from build123d import *

# Parameters (mm, degrees)
F1_DEPTH  = 25.4
F2_W      = 9.525
F2_H      = 19.05
F3_DEPTH  = 134.62
F4_W      = 9.525
F4_H      = 19.05
F5_DEPTH  = 157.48
F6_R      = 1.651
F7_DEPTH  = 25.4
F8_W      = 25.4
F8_H      = 7.62
F9_DEPTH  = 101.6
F10_W     = 15.24
F10_H     = 19.05
F10_W_2   = 25.4
F11_DEPTH = 25.4
F12_W     = 38.1
F12_H     = 18.161
F13_DEPTH = 25.4


with BuildPart() as f1:
    # F0 (on Top) → F1 (new body)
    with BuildSketch(Plane.XY):
        Polygon((125.723586, 125.723586), (0, 0), (152.4, 0), (152.4, 12.7), (31.75, 12.7), (135.248586, 116.198586), align=None)
    extrude(amount=F1_DEPTH)

    # F2 (on face) → F3 (cut)
    with BuildSketch(Plane.YZ.offset(152.4)):
        with Locations((7.9375, 12.7)):
            Rectangle(F2_W, F2_H)
    extrude(amount=-F3_DEPTH, mode=Mode.SUBTRACT)

    # F4 (on face) → F5 (cut)
    with BuildSketch(Plane(origin=(125.723586, 125.723586, 0), x_dir=(-0.707107, 0.707107, 0), z_dir=(0.707107, 0.707107, 0))):
        with Locations((-8.707884, 12.7)):
            Rectangle(F4_W, F4_H)
    extrude(amount=-F5_DEPTH, mode=Mode.SUBTRACT)

    # F6 (on face) → F7 (cut)
    with BuildSketch(Plane(origin=(0, 3.175, 0), x_dir=(-1, 0, 0), z_dir=(0, 1, 0))):
        with Locations((-88.9, 12.7)):
            Circle(F6_R)
        with Locations((-50.8, 12.7)):
            Circle(F6_R)
        with Locations((-127, 12.7)):
            Circle(F6_R)
    extrude(amount=-F7_DEPTH, mode=Mode.SUBTRACT)

    # F8 (on face) → F9 (cut)
    with BuildSketch(Plane.XY.offset(25.4)):
        with Locations((38.1, 6.35)):
            Rectangle(F8_W, F8_H)
        with Locations((69.85, 6.35)):
            Rectangle(F8_W, F8_H)
        with Locations((101.6, 6.35)):
            Rectangle(F8_W, F8_H)
        with Locations((133.35, 6.35)):
            Rectangle(F8_W, F8_H)
        Polygon((128.962406, 113.504509), (122.676227, 119.790688), (104.715715, 101.830176), (111.001894, 95.543997), align=None)
        Polygon((106.865048, 90.700587), (100.578869, 96.986766), (82.618356, 79.026254), (88.904536, 72.740075), align=None)
        Polygon((84.061126, 68.603228), (77.774947, 74.889408), (59.814434, 56.928895), (66.100614, 50.642716), align=None)
        Polygon((61.755537, 46.007537), (55.469357, 52.293716), (37.508845, 34.333204), (43.795024, 28.047025), align=None)
    extrude(amount=-F9_DEPTH, mode=Mode.SUBTRACT)

    # F10 (on face) → F11 (cut)
    with BuildSketch(Plane.XZ):
        with Locations((138.455176, 12.7)):
            Rectangle(F10_W, F10_H)
        with Locations((106.998765, 12.7)):
            Rectangle(F10_W_2, F10_H)
        with Locations((68.713241, 12.7)):
            Rectangle(F10_W_2, F10_H)
        with Locations((33.749367, 12.7)):
            Rectangle(F10_W_2, F10_H)
    extrude(amount=-F11_DEPTH, mode=Mode.SUBTRACT)

    # F12 (on face) → F13 (cut)
    with BuildSketch(Plane(origin=(0, 0, 0), x_dir=(-0.707107, -0.707107, 0), z_dir=(-0.707107, 0.707107, 0))):
        with Locations((-108.820044, 12.337992)):
            Rectangle(F12_W, F12_H)
        with Locations((-152.4, 12.337992)):
            Rectangle(F12_W, F12_H)
        with Locations((-64.913327, 12.337992)):
            Rectangle(F12_W, F12_H)
    extrude(amount=-F13_DEPTH, mode=Mode.SUBTRACT)


solid = f1.part
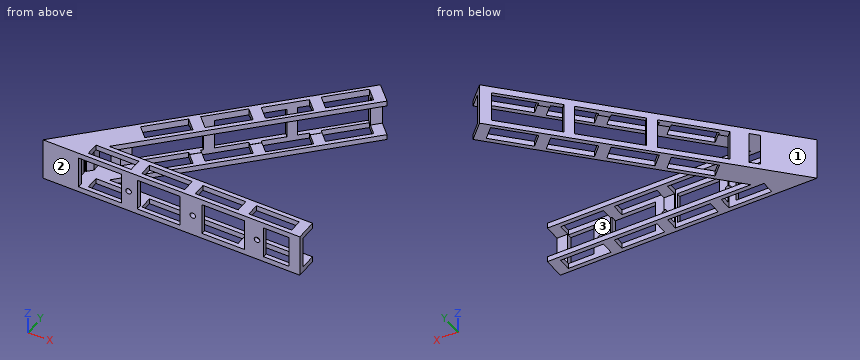
Geometry check sheet. Reference: the model listing, model coordinates, mm. Face numbers are marked on the shaded views. Coordinates: 2 decimals unless noted, no trailing zeros. Use a Markdown table: item, result. Add a question column.
1. Go/stop test with flat-tipped pins: pin 1 Ø3 at (y, z) = (17, 14) entering from +X; pin 2 Ø1.5 at (y, z) = (30.5, 19) entering from +X; pin 3 Ø2.5 at (y, z) = (5.5, 23.5) entering from -X; pin 4 Ø2 at (x, y) = (71.5, 73.5) entering from +Z. Record where each tip stops, or that it passes through.
2. Cross-section at A-A (y = 38.5). Give the number of separate pieces and of enclosed holes in the cut face, and give its area (3 significant figures).
3. Material ranges on L1, parallel to Z at x = 88.9, y = 2.35; L2, parallel to Y at x = 78, z = 23.25; L3, parallel to Z at x = 88, y = 1, recorded low to high.
4. Mould release check, pull along X, two halves, no side actions. Record for the marked faces 1, 2 and 3: pulls with the +X half, pulls with the -X half, needs draft (parallel to the pull), parting line crosses it, or undercut.
Filled sheet:
| question | item | result |
|---|---|---|
| 1 | pin 1 | x = 21.05 |
| 1 | pin 2 | x = 35.11 |
| 1 | pin 3 | x = 4.25 |
| 1 | pin 4 | through |
| 2 | separate pieces | 4 |
| 2 | enclosed holes | 0 |
| 2 | area | 44.0 mm2 |
| 3 | L1 | 0 to 11.05, 14.35 to 25.4 |
| 3 | L2 | 0 to 2.54, 10.16 to 12.7, 58.95 to 62.54, 74.66 to 78 |
| 3 | L3 | 0 to 11.32, 14.08 to 25.4 |
| 4 | face 1 | pulls with the -X half |
| 4 | face 2 | needs draft |
| 4 | face 3 | undercut |
